Autodesk Inventor part; units mm, degrees
ref_plane "YZ Plane" through (0, 0, 0) normal (1, 0, 0) x (0, 1, 0)
ref_plane "XZ Plane" through (0, 0, 0) normal (0, 1, 0) x (-1, 0, 0)
ref_plane "XY Plane" through (0, 0, 0) normal (0, 0, 1) x (1, 0, 0)
sketch "スケッチ1" plane through (0, 0, 0) normal (0, 0, 1) x (1, 0, 0)
  circle A0 centre (-4.0763, -4.0763) radius 35.7
  circle A1 centre (-4.0763, -4.0763) radius 35.7
  circle A2 centre (-33.3097, 3.7568) radius 2.1
  circle A3 centre (3.7568, -33.3097) radius 2.1
  circle A4 centre (17.3241, 17.3241) radius 2.1
  dimension "d0" = 4.2
  dimension "d1" = 4.2
  dimension "d2" = 4.2
  dimension "d3" = 71.4
extrude "押し出し1" add sketch "スケッチ1" along normal blind 5
sketch "スケッチ3" plane through (-4.0763, -4.0763, 0) normal (0, 0, -1) x (-1, 0, 0)
  circle A0 centre (0, 0) radius 10.5
  circle A1 centre (-6.092, 6.092) radius 1.2385
  circle A2 centre (-8.6154, 0) radius 1.2385
  circle A3 centre (-6.092, -6.092) radius 1.2385
  circle A4 centre (0, -8.6154) radius 1.2385
  circle A5 centre (6.092, -6.092) radius 1.2385
  circle A6 centre (0, 8.6154) radius 1.2385
  circle A7 centre (6.092, 6.092) radius 1.2385
  circle A8 centre (8.6154, 0) radius 1.2385
  circle A9 centre (0, 0) radius 5.9231
  point P0 (-4.0763, 4.0763)
  dimension "d12" = 21
extrude "押し出し3" add sketch "スケッチ3" along normal blind 5.5
properties part number "rotate_plate_2"
Input: part model. Units: mm. Frame: model coordinates. A direction names the side the tool comes from. Give positions to 0.01 mm unless a question says otherwise; leave off trailing zeros. Order: outer loops, then holes, each group sorted by start corner. A loop starts at its lowest first (then second) coordinate and runs counter-clockwise, first axis right, second up. Notation, with made-up numbers: M 79,-26 L 88,-26 A28 cw 88,13 Z; hole C 57,62 d10. An arc over 180 degrees is marked long. One line per question, with ' | ' between items. Start each with the question number.
1. Section query D-D (y = -2). Return the cut outline in (x, z).
2. Pull-direction query (X, two-part tool) for faces 1 (the face through (-8.92, 5.24, -2.71)), 2 (the face through (-5, -4, 5)), 3 (the face through (-9.55, -1.81, -2.71)); classes: released by +X, released by -X, zero draft, split by the parting line, or undercut.
3. Section query B-B (z = -3.25). Count the separate pieces of the cut face and the enclosed holes in it, and give its area (3 significant figures).
4. Access query for faces 4 (the face through (-10, -10, 0)), 5 (the face through (4.73, -31.45, 2.46)). Directions: +Z, -Z, +X, -X, +Y, -Y. A direction counts if a zero-diameter tool reaches every point of the face in a straight line with its end or side. Return the directions, or none.
5. First-contact query: pin 1 Ø4 at (x, y) = (-10.17, 2.02) entering from -Z; pin 2 Ø2 at (x, z) = (-32.5, 1.5) entering from -Y; pin 3 Ø1 at (x, z) = (-10.5, 2) entering from +Y; pin 4 Ø2 at (x, y) = (2.02, -10.17) entering from -Z. Flat tips, straight axial feed; report the tip coordinate or a pass-through.
6. Material intervals for probe 1 along Z at (x, y) = (26, 14); probe 2 along Y at (x, z) = (1, -1.25); probe 3 along X at (y, z) = (-12, -4.5), sorted ascending. Write a range as [from, to].
7. Section query C-C (y = 16.5). Return the cut outline in (x, z), and give its area (3 significant figures).
8. Section query A-A (x = 17). Return the cut outline in (y, z), and give its area (3 significant figures).
Here are the results:
1) outline: M -39.72,0 L -14.37,0 L -14.37,-5.5 L -9.62,-5.5 L -9.62,0 L 1.47,0 L 1.47,-5.5 L 6.22,-5.5 L 6.22,0 L 31.56,0 L 31.56,5 L -39.72,5 Z
2) face 1: split by the parting line | face 2: zero draft | face 3: undercut
3) separate pieces: 1 | enclosed holes: 9 | area: 198 mm²
4) face 4: -Z | face 5: +Z, -Z
5) pin 1: z = -5.5 | pin 2: y = -26.93 | pin 3: y = 31.13 | pin 4: z = 0
6) probe 1: [0, 5] | probe 2: [-13.27, -10.88], [-9.46, -7.13], [-1.02, 1.31], [2.72, 5.12] | probe 3: [-10.97, -5.1], [-3.05, 2.81]
7) outline: M -33.25,0 L 15.39,0 L 15.39,5 L -33.25,5 Z; M 19.26,0 L 25.1,0 L 25.1,5 L 19.26,5 Z | area: 272 mm²
8) outline: M -32.89,0 L 15.25,0 L 15.25,5 L -32.89,5 Z; M 19.4,0 L 24.74,0 L 24.74,5 L 19.4,5 Z | area: 267 mm²
